Geometry check sheet. Reference: the model listing, model coordinates, mm. A direction names the side the tool comes from. Coordinates: 2 decimals unless noted, no trailing zeros. Write each loop counter-clockwise with the first axis right and the second up, starting at its lowest first coordinate (ties: lowest second). Pieces come first, ordered by that corner, then holes. Notation, with made-up numbers: M 55.5,-33.75 L 102.5,-33.75 A35 cw 102.5,5.25 Z; hole C -25,-9.75 d6. An arc over 180 degrees is marked long. Put each result on its own line as item: value. Start each with the question number.
1) Cross-section at D-D on z = 37. Record the cut outline in (x, y), plus the area to 3 significant figures.
2) Gauge pin test, flat ends, axial feed: pin 1 (4 mm diameter, centred on x = 0, y = 0, fed in from -Z); pin 2 (5 mm diameter, centred on y = -6, z = 32, fed in from -X); pin 3 (1.5 mm diameter, centred on x = 2, z = 27, fed in from +Y). Record the tip position at first contact, or that the pin passes through.
3) Set-up check for faces 4 (the cylindrical face through (-0.708, -3.186, -35.496)), 5 (the flat face through (3, -2, -45.669)), 6 (the cylindrical face through (0.708, -3.186, 35.496)): record each of +Z, -Z, +X, -X, +Y, -Y from which the full face is reachable in a straight line by a thin tool's end or side.
4) Mould release check, pull along X, two halves, no side actions. Record for faces 1 (the cylindrical face through (-1.032, 7.857, -31.582)), 2 (the conical face through (0.07, 0.56, -23.98)), 3 (the flat face through (3, -2, 45.669)): released by +X, released by -X, zero draft, split by the parting line, or undercut.
5) Scan lines: line 1 along Y through (x, z) = (0, 31.75); line 2 along Y through (x, z) = (2, 31.5); line 3 along X through (y, z) = (1, 37). Record each from-to range of solid material in increasing order.
6) Cross-section at C-C on z = -4.5. Record the cut outline in (x, y) (1 decimal), plus the area to 3 significant figures.
from build123d import *

# Parameters (mm, degrees)
SKETCH1_R                    = 7.9375
EXTRUDE1_DEPTH               = 45.6692
F_5_16_18_TAPPED_HOLE1_D     = 6.5278
F_5_16_18_TAPPED_HOLE1_DEPTH = 20.066
F_5_16_18_TAPPED_HOLE1_TIP   = 1.961148974
F_5_16_18_TAPPED_HOLE2_D     = 6.5278
F_5_16_18_TAPPED_HOLE2_DEPTH = 20.066
F_5_16_18_TAPPED_HOLE2_TIP   = 1.961148974
SKETCH6_R                    = 7.9375
SKETCH6_R_2                  = 7.9248
CUT_EXTRUDE1_DEPTH           = 28.575


with BuildPart() as part:
    # Sketch1 → Extrude1 (new body, symmetric)
    with BuildSketch(Plane.XY):
        Circle(SKETCH1_R)
    extrude(amount=EXTRUDE1_DEPTH, both=True)

    # 5/16-18 Tapped Hole1
    with Locations(Plane.XY.offset(45.6692)):
        with Locations((0, 0)):
            Hole(F_5_16_18_TAPPED_HOLE1_D / 2, depth=F_5_16_18_TAPPED_HOLE1_DEPTH)
            with Locations((0, 0, -(F_5_16_18_TAPPED_HOLE1_DEPTH + F_5_16_18_TAPPED_HOLE1_TIP / 2))):  # 118° drill point
                Cone(0, F_5_16_18_TAPPED_HOLE1_D / 2, F_5_16_18_TAPPED_HOLE1_TIP, mode=Mode.SUBTRACT)

    # 5/16-18 Tapped Hole2
    with Locations(Plane(origin=(0, 0, -45.6692), x_dir=(-1, 0, 0), z_dir=(0, 0, -1))):
        with Locations((0, 0)):
            Hole(F_5_16_18_TAPPED_HOLE2_D / 2, depth=F_5_16_18_TAPPED_HOLE2_DEPTH)
            with Locations((0, 0, -(F_5_16_18_TAPPED_HOLE2_DEPTH + F_5_16_18_TAPPED_HOLE2_TIP / 2))):  # 118° drill point
                Cone(0, F_5_16_18_TAPPED_HOLE2_D / 2, F_5_16_18_TAPPED_HOLE2_TIP, mode=Mode.SUBTRACT)

    # Sketch6 → Cut-Extrude1 (cut)
    with BuildSketch(Plane.XY.offset(45.6692)):
        Circle(SKETCH6_R)
        Circle(SKETCH6_R_2, mode=Mode.SUBTRACT)
    cut_extrude1 = extrude(amount=-CUT_EXTRUDE1_DEPTH, mode=Mode.SUBTRACT)

    # Mirror1: Cut-Extrude1 across plane
    add(cut_extrude1.mirror(Plane.XY), mode=Mode.SUBTRACT)


solid = part.part
Answer key:
1. outline: C 0,0 d15.85; hole C 0,0 d6.53
1. area: 164 mm²
2. pin 1: stops at z = -24.84
2. pin 2: stops at x = -7.11
2. pin 3: stops at y = 7.83
3. face 4: -Z
3. face 5: -Z, +X, -X, +Y, -Y
3. face 6: +Z
4. face 1: split by the parting line
4. face 2: undercut
4. face 3: zero draft
5. line 1: y = -7.92 to -3.26, 3.26 to 7.92
5. line 2: y = -7.67 to -2.58, 2.58 to 7.67
5. line 3: x = -7.86 to -3.11, 3.11 to 7.86
6. outline: C 0,0 d15.9
6. area: 198 mm²
